Can you work these out from the drawing? Everything is in mm from the part's minimum corner. Coordinates: 2 decimals unless noted, no trailing zeros. Order: outer loops, then holes, each group sorted by start corner. A loop starts at its lowest first (then second) coordinate and runs counter-clockwise, first axis right, second up. Notation, with made-up numbers: (65.5, 71.5) -> (124.5, 71.5) arc R25 cw to (124.5, 99.5) -> close; hole circle Ø6 at (74.25, 71.25). An arc over 180 degrees is marked (long way). Answer in a Markdown table with one row per item.
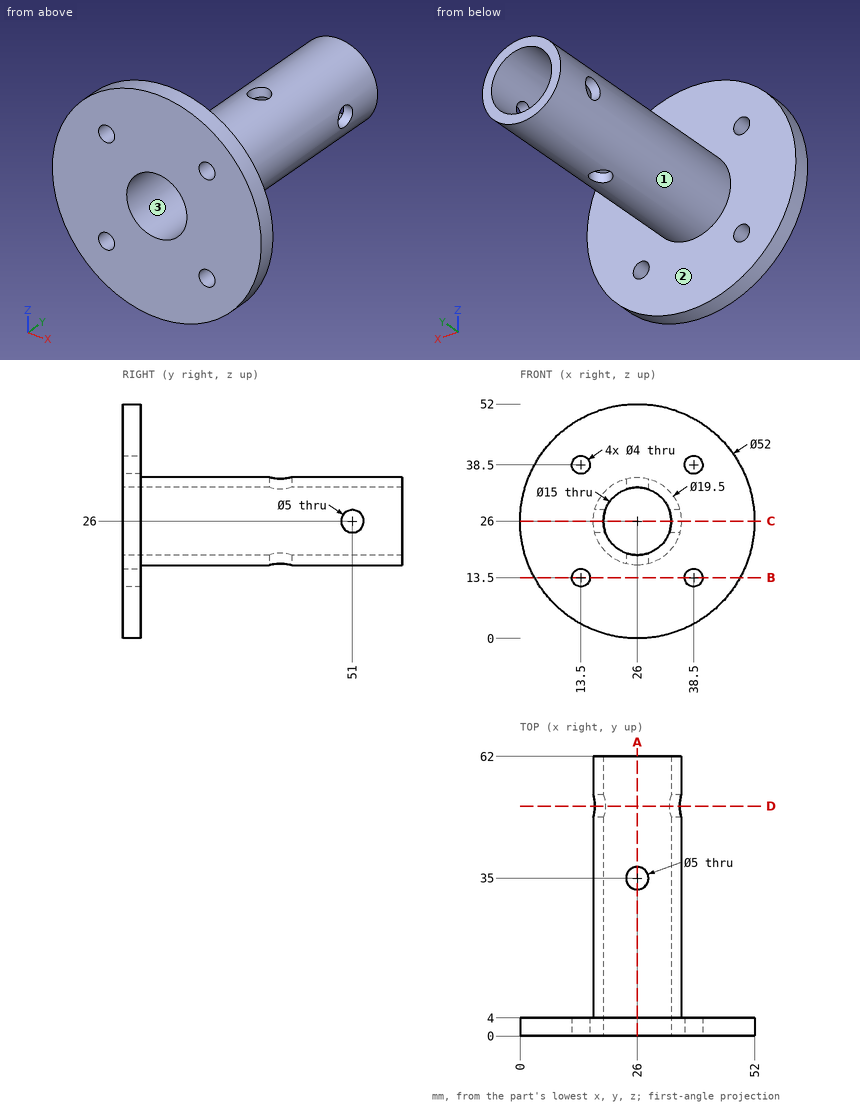
(1) We'd pull the mould along Z, two halves only. Please class the marked faces 1, 2 and 3: +Z half, -Z half, draft (parallel to the pull), parting line (faces both ways), or undercut.
Response values:
| item | result |
|---|---|
| face 1 | parting line |
| face 2 | draft |
| face 3 | undercut |
(2) Suppose I cut it at A-A (x = 26). Please give me the cut outline in (y, z).
Response values:
| item | result |
|---|---|
| outline | (0, 0) -> (4, 0) -> (4, 16.25) -> (32.5, 16.25) -> (32.5, 18.5) -> (0, 18.5) -> close; (0, 33.5) -> (32.5, 33.5) -> (32.5, 35.75) -> (4, 35.75) -> (4, 52) -> (0, 52) -> close; (37.5, 16.25) -> (62, 16.25) -> (62, 18.5) -> (37.5, 18.5) -> close; (37.5, 33.5) -> (62, 33.5) -> (62, 35.75) -> (37.5, 35.75) -> close |
(3) Will these pins go through, and if not, where does the flat tip stop? pin 1 Ø3 at (x, y) = (26, 35) entering from -Z; pin 2 Ø8 at (y, z) = (51.5, 17) entering from -X; pin 3 Ø1.5 at (x, z) = (13.5, 18) entering from +Y; pin 4 Ø8 at (y, z) = (44, 37.5) entering from -X.
Response values:
| item | result |
|---|---|
| pin 1 | through |
| pin 2 | x = 17.63 |
| pin 3 | y = 4 |
| pin 4 | x = 19.77 |
(4) Suppose I cut it at D-D (y = 51). Please give me the cut outline in (x, z).
Response values:
| item | result |
|---|---|
| outline | (16.58, 23.5) arc R9.75 ccw to (35.42, 23.5) -> (33.07, 23.5) arc R7.5 cw to (18.93, 23.5) -> close; (16.58, 28.5) -> (18.93, 28.5) arc R7.5 cw to (33.07, 28.5) -> (35.42, 28.5) arc R9.75 ccw to start |
(5) I need wall thicknesses on line 1 (X direction, y = 38, z = 26); line 2 (Y direction, x = 39.5, z = 24); line 3 (Y direction, x = 17.75, z = 26). Which ranges of each line are inside material? Lowest first, please. Write a range as [from, to].
Response values:
| item | result |
|---|---|
| line 1 | [16.25, 18.5], [33.5, 35.75] |
| line 2 | [0, 4] |
| line 3 | [0, 48.5], [53.5, 62] |
(6) Suppose I cut it at B-B (z = 13.5). Please give me the cut outline in (x, y).
Response values:
| item | result |
|---|---|
| outline | (3.2, 0) -> (11.5, 0) -> (11.5, 4) -> (3.2, 4) -> close; (15.5, 0) -> (36.5, 0) -> (36.5, 4) -> (15.5, 4) -> close; (40.5, 0) -> (48.8, 0) -> (48.8, 4) -> (40.5, 4) -> close |
(7) Suppose I cut it at C-C (z = 26). Please give me the cut outline in (x, y).
Response values:
| item | result |
|---|---|
| outline | (0, 0) -> (18.5, 0) -> (18.5, 48.5) -> (16.25, 48.5) -> (16.25, 4) -> (0, 4) -> close; (16.25, 53.5) -> (18.5, 53.5) -> (18.5, 62) -> (16.25, 62) -> close; (33.5, 0) -> (52, 0) -> (52, 4) -> (35.75, 4) -> (35.75, 48.5) -> (33.5, 48.5) -> close; (33.5, 53.5) -> (35.75, 53.5) -> (35.75, 62) -> (33.5, 62) -> close |
